Check sheet for the drawn part. Datum: minimum x, y, z corner. Units: mm. A direction names the side the tool comes from. Coordinates: 2 decimals unless noted, no trailing zeros. Order: outer loops, then holes, each group sorted by start corner. A loop starts at its lowest first (then second) coordinate and runs counter-clockwise, first axis right, second up.
1. Cross-section at C-C (x = 66). Enter the section's corners in (y, z), then the cut area to 3 significant figures.
2. Cross-section at D-D (z = 151.5). Enter the section's corners in (x, y), then the cut area to 3 significant figures.
3. Draft check along X on the marked faces 3, 4, 5 and 6. Enter one of: released by +X, released by -X, zero draft, split by the parting line, or undercut.
4. Thickness scan on line 1 (Z direction, x = 275, y = 29); line 2 (X direction, y = 15, z = 25); line 3 (X direction, y = 26.5, z = 153). Record the ranges inside material, lowest first.
5. Gauge pin test, flat ends, axial feed: pin 1 Ø10 at (y, z) = (56, 74.5) entering from +X; pin 2 Ø3 at (x, z) = (266.5, 152.5) entering from +Y; pin 3 Ø6 at (y, z) = (56, 67) entering from -X. Record the tip position at first contact, or that the pin passes through.
6. Cross-section at A-A (y = 20). Enter the section's corners in (x, z), then the cut area to 3 significant figures.
7. Set-up check for the marked faces 1 and 2: record each of +Z, -Z, +X, -X, +Y, -Y from which the full face is reachable in a straight line by a thin tool's end or side.
8. Cross-section at B-B (z = 62.5). Enter the section's corners in (x, y).
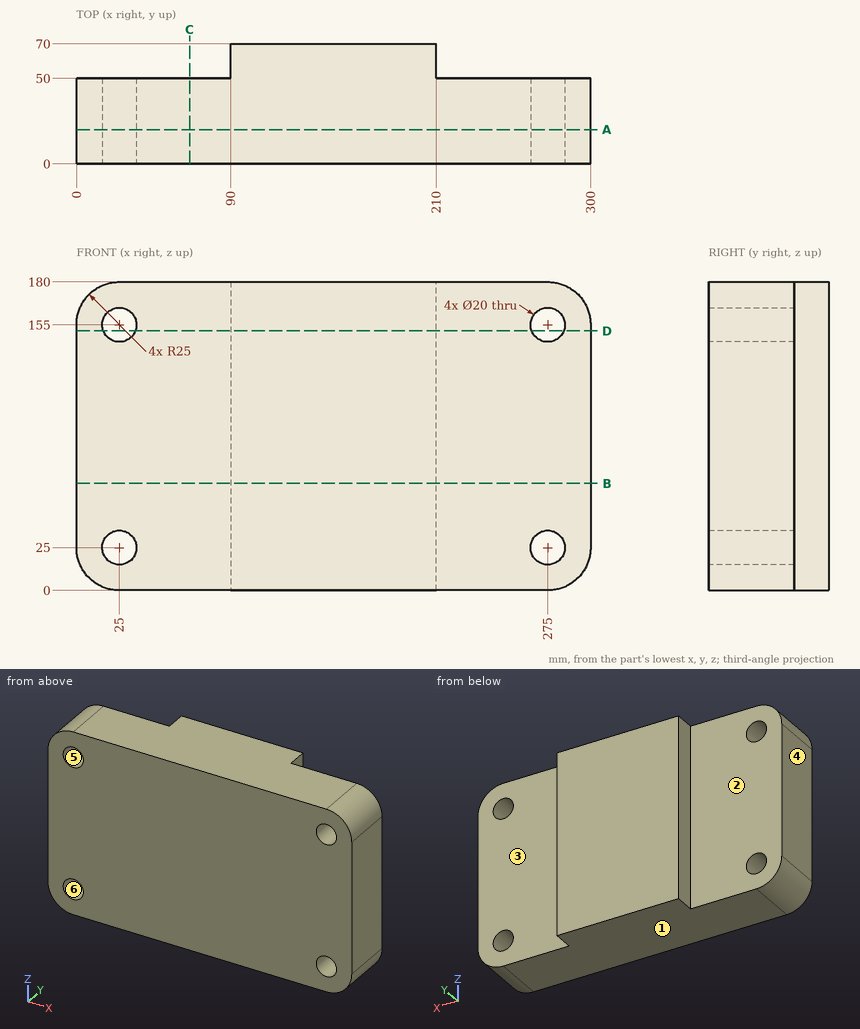
Data:
1. outline: (0, 0) - (50, 0) - (50, 180) - (0, 180) - close
1. area: 9,000 mm2
2. outline: (0, 0) - (15.63, 0) - (15.63, 50) - (0, 50) - close; (34.37, 0) - (265.63, 0) - (265.63, 50) - (210, 50) - (210, 70) - (90, 70) - (90, 50) - (34.37, 50) - close; (284.37, 0) - (300, 0) - (300, 50) - (284.37, 50) - close
2. area: 15,500 mm2
3. face 3: zero draft
3. face 4: released by -X
3. face 5: undercut
3. face 6: undercut
4. line 1: z = 0 to 15, 35 to 145, 165 to 180
4. line 2: x = 0 to 15, 35 to 265, 285 to 300
4. line 3: x = 0 to 15.2, 34.8 to 265.2, 284.8 to 300
5. pin 1: stops at x = 210
5. pin 2: stops at y = 50
5. pin 3: stops at x = 90
6. outline: (0, 25) arc R25 ccw to (25, 0) - (275, 0) arc R25 ccw to (300, 25) - (300, 155) arc R25 ccw to (275, 180) - (25, 180) arc R25 ccw to (0, 155) - close; hole circle Ø20 at (25, 25); hole circle Ø20 at (25, 155); hole circle Ø20 at (275, 25); hole circle Ø20 at (275, 155)
6. area: 52,200 mm2
7. face 1: -Z, +X, -X, +Y, -Y
7. face 2: +Z, -Z, -X, +Y
8. outline: (0, 0) - (300, 0) - (300, 50) - (210, 50) - (210, 70) - (90, 70) - (90, 50) - (0, 50) - close
